Design review of the part built by this model. Coordinates are the model's own, in mm. Face numbers are marked on the shaded views. A direction names the side the tool comes from. Give positions to 0.01 mm unless a question says otherwise; leave off trailing zeros. Write each loop counter-clockwise with the first axis right and the second up, starting at its lowest first coordinate (ties: lowest second). Pieces come first, ordered by that corner, then holes. Notation, with made-up numbers: (38, 56) -> (61, 56) arc R33 cw to (61, 93) -> close; hole circle Ø11 at (75.5, 31.5). An arc over 180 degrees is marked (long way). Put each result on its own line as item: value. Start each with the question number.
Autodesk Inventor part; units mm, degrees
ref_plane "Work Plane6" through (29.6406, -20.7378, 44) normal (0, 0, 1) x (1, 0, 0)
ref_plane "YZ Plane" through (0, 0, 0) normal (1, 0, 0) x (0, 1, 0)
ref_plane "XZ Plane" through (0, 0, 0) normal (0, 1, 0) x (-1, 0, 0)
ref_plane "Work Plane1" through (0, 0, 0) normal (0, 0, 1) x (1, 0, 0)
sketch "Sketch1" plane through (0, 0, 0) normal (0, 0, 1) x (1, 0, 0)
  circle A0 centre (7.5, 0) radius 3.175
  circle A1 centre (7.5, 15) radius 2.5 construction
  circle A2 centre (7.5, -15) radius 2.5 construction
  arc A3 (69.3283, 4.3421) -> (-40.362, 3.8938) centre (14.5, 0) ccw construction
  arc A4 (17.9696, 54.8905) -> (17.9696, -54.8905) centre (7.5, 0) ccw
  arc A5 (60.9943, -59.4841) -> (60.9943, 59.4841) centre (7.5, 0) ccw
  line L0 (60.9943, 59.4841) -> (17.9696, 54.8905)
  line L1 (60.9943, -59.4841) -> (17.9696, -54.8905)
  point P0 (0, 0)
  dimension "d0" = 55.88
extrude "Primary Shaft Bore" add sketch "Sketch1" along normal blind 5
sketch "Sketch2" plane through (0, 0, 5) normal (0, 0, 1) x (1, 0, 0)
  circle A0 centre (7.5, 0) radius 3.175 construction
  circle A1 centre (7.5, 0) radius 3.175
  circle A2 centre (7.5, 0) radius 20.32
  circle A3 centre (7.5, 0) radius 21.59
  point P0 (0, 0)
  dimension "d3" = 40.64
  dimension "d4" = 43.18
extrude "Large Gear Seat" add sketch "Sketch2" along normal blind 5 contours A3
sketch "Sketch4" plane through (0, 0, 0) normal (0, 0, -1) x (-1, 0, 0)
  circle A0 centre (-7.5, 15) radius 2.5 construction
  circle A1 centre (-7.5, -15) radius 2.5 construction
  point P0 (0, 0)
ref_plane "Work Plane2" through (-496.14, 0, 5) normal (0, 1, 0) x (0, 0, -1)
sketch "Sketch5" plane through (0, 0, 5) normal (0, 0, 1) x (1, 0, 0)
  circle A0 centre (7.5, 0) radius 3.175
  circle A1 centre (7.5, 15) radius 1.5
  circle A2 centre (7.5, -15) radius 1.5
  point P0 (0, 0)
ref_plane "Work Plane5" through (7.5, 0, 5) normal (-1, 0, 0) x (0, -1, 0)
sketch "Sketch7" plane through (0, 0, 5) normal (0, 0, 1) x (1, 0, 0)
  arc A0 (51.7179, -2) -> (48.3952, -2) centre (50.0565, 0) ccw construction
  circle A1 centre (50.0565, 0) radius 6.985
  point P0 (0, 0)
  dimension "d17" = 13.97
extrude "Second Gear Seat" add sketch "Sketch7" along normal up to surface (5 mm away)
sketch "Sketch8" plane through (0, 0, 5) normal (0, 0, 1) x (1, 0, 0)
  point P0 (0, 0)
  point P1 (7.5, 15)
  point P2 (7.5, -15)
hole "Hole1" at (7.5, 15, 5) at (7.5, -15, 5) direction (0, 0, -1) diameter 4.4958 end through all counterbore diameter 9.398 counterbore depth 1.5875
sketch "Sketch9" plane through (50.0565, 0, 10) normal (0, 0, 1) x (1, 0, 0)
  arc A0 (1.6613, -2) -> (-1.6613, -2) centre (0, 0) ccw construction
  circle A1 centre (0, 0) radius 2.75
  point P0 (-50.0565, 0)
  dimension "d27" = 5.5
extrude "Extrusion7" cut sketch "Sketch9" against normal blind 6
sketch "Sketch10" plane through (0, 0, 5) normal (0, 0, 1) x (1, 0, 0)
  line L0 (114.676, 0) -> (-75.556, 0) construction
  line L1 (71.4406, -11.5878) -> (71.4406, 11.4122) construction
  line L2 (61.7906, 21.0622) -> (38.7906, 21.0622) construction
  line L3 (38.7906, -21.2378) -> (61.7906, -21.2378) construction
  line L4 (67.587, -21.0914) -> (71.2941, -17.3843) construction
  line L5 (71.2941, 17.2086) -> (67.587, 20.9157) construction
  line L6 (39.7906, -21.4378) -> (68.6548, -21.4378)
  line L7 (68.6548, -21.4378) -> (71.5406, -18.552)
  line L8 (71.5406, -18.552) -> (71.5406, 0)
  line L9 (39.7906, -21.4378) -> (39.7906, -26.4378)
  line L10 (39.7906, -26.4378) -> (76.5406, -26.4378)
  line L11 (76.5406, -26.4378) -> (76.5406, 0)
  line L12 (39.7906, 21.4378) -> (68.6548, 21.4378)
  line L13 (68.6548, 21.4378) -> (71.5406, 18.552)
  line L14 (71.5406, 18.552) -> (71.5406, 0)
  line L15 (39.7906, 21.4378) -> (39.7906, 26.4378)
  line L16 (39.7906, 26.4378) -> (76.5406, 26.4378)
  line L17 (76.5406, 26.4378) -> (76.5406, 0)
  point P0 (0, 0)
  dimension "d30" = 0.2
  dimension "d31" = 0.1
  dimension "d32" = 5
  dimension "d33" = 5
  dimension "d34" = 1
  dimension "d35" = 1
ref_plane "Work Plane6" through (29.6406, -20.7378, 44) normal (0, 0, 1) x (1, 0, 0)
extrude "Extrusion8" add sketch "Sketch10" along normal up to surface (39 mm away)
sketch "Sketch11" plane through (71.5406, -18.552, 5) normal (-1, 0, 0) x (0, 0, 1)
  line L0 (0, -2.8858) -> (39, -2.8858)
  line L1 (18.9, -2.8858) -> (16.36, -2.8858)
  line L2 (16.36, -2.8858) -> (16.36, 40.2564)
  line L3 (16.36, 40.2564) -> (18.9, 40.2564)
  line L4 (18.9, 40.2564) -> (18.9, -2.8858)
  line L5 (19, 35.4071) -> (19, 1.5213) construction
  point P0 (-5, 18.552)
  dimension "d38" = 2.54
  dimension "d39" = 0.1
extrude "Extrusion9" add sketch "Sketch11" along normal blind 10.16
sketch "Sketch12" plane through (0, 0, 0) normal (0, 0, -1) x (-1, 0, 0)
  line L0 (-61.3806, 21.4378) -> (-61.3806, -21.4378)
  line L1 (-39.7906, -21.4378) -> (-68.6548, -21.4378)
  line L2 (-68.6548, -21.4378) -> (-71.5406, -18.552)
  line L3 (-71.5406, -18.552) -> (-71.5406, 18.552)
  line L4 (-71.5406, 18.552) -> (-68.6548, 21.4378)
  line L5 (-68.6548, 21.4378) -> (-39.7906, 21.4378)
  point P0 (0, 0)
extrude "Extrusion10" cut sketch "Sketch12" against normal blind 10.16
sketch "Sketch13" plane through (71.5406, -18.552, 21.36) normal (0, 0, -1) x (-1, 0, 0)
  circle A0 centre (5.75, 2.9642) radius 2.4 construction
  circle A1 centre (5.75, 33.9642) radius 2.4 construction
  point P0 (71.5406, 18.552)
hole "Hole2" at (65.7906, -15.5878, 21.36) at (65.7906, 15.4122, 21.36) direction (0, 0, 1) diameter 3.4036 end through all countersink diameter 6.2992 countersink angle 90
properties part number "TopGearPlate"
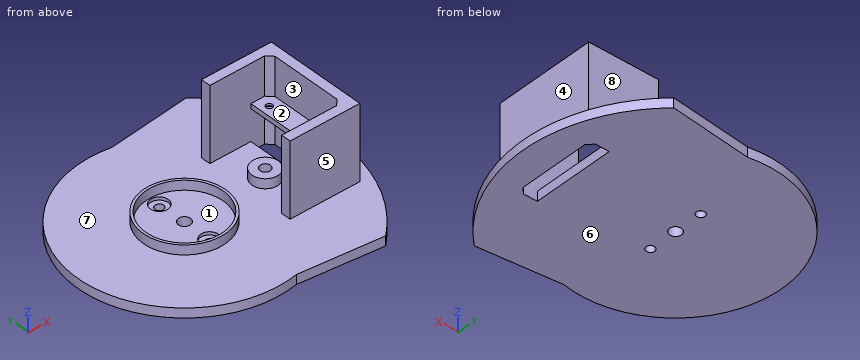
Q1. Take a section at A-A on x = 7.5. State how many separate pieces and enclosed holes the cut face has, then the cut area to 3 significant figures.
Q2. Mouldability with a two-part tool opening along X and no side actions: class the marked faces 1, 2 and 3 as +X half, -X half, draft (parallel to the pull), parting line (faces both ways), or undercut.
Q3. Take a section at C-C on z = 12.5. Give the boundary of the cut face in (x, y).
Q4. To check wall thickness, follow probe 1 along Y at (x, z) = (61, 36); probe 2 along X at (y, z) = (-15, 4.6); probe 3 along Z at (x, y) = (57, -43). State the ranges of each line that lie inside material, in increasing order. Write a range as from..to.
Q5. Take a section at D-D on x = -9. Give the boundary of the cut face in (y, z).
Q6. For pin 1 (18.5 mm diameter, centred on x = 63.5, z = 28.5, fed in from -Y); pin 2 (21.5 mm diameter, centred on x = 12, y = 7, fed in from +Z); pin 3 (2.5 mm diameter, centred on x = 65.79, y = -15.59, fed in from +Z); pin 4 (12 mm diameter, centred on x = 48.5, z = 6.5, fed in from -Y), all flat-tipped, find the tip position at first contact; note any pin that passes through.
Q7. Machinability: for the marked faces 4, 5, 6, 7 and 8, which of the approach directions +Z, -Z, +X, -X, +Y, -Y give a long, thin tool a straight path to every point of the face, cutting with its end or side? Answer none if there is none.
Result:
1. separate pieces: 4
1. enclosed holes: 0
1. area: 479 mm^2
2. face 1: undercut
2. face 2: draft
2. face 3: -X half
3. outline: (39.79, -26.44) -> (76.54, -26.44) -> (76.54, 26.44) -> (39.79, 26.44) -> (39.79, 21.44) -> (68.65, 21.44) -> (71.54, 18.55) -> (71.54, -18.55) -> (68.65, -21.44) -> (39.79, -21.44) -> close
4. probe 1: y = -26.44..-21.44, 21.44..26.44
4. probe 2: x = -46.33..2.8, 12.2..61.38, 71.54..86.08
4. probe 3: z = 0..5
5. outline: (-53.39, 0) -> (53.39, 0) -> (53.39, 5) -> (13.92, 5) -> (13.92, 10) -> (11.86, 10) -> (11.86, 5) -> (-11.86, 5) -> (-11.86, 10) -> (-13.92, 10) -> (-13.92, 5) -> (-53.39, 5) -> close
6. pin 1: stops at y = -26.44
6. pin 2: stops at z = 5
6. pin 3: passes through
6. pin 4: stops at y = -58.77
7. face 4: +Z, +X, +Y, -Y
7. face 5: +Z, +X, -X, -Y
7. face 6: -Z, +X, -X, +Y, -Y
7. face 7: +Z
7. face 8: +Z, +X, -X, +Y
